Study the drawing (mm; zero at the part's minimum x, y, z) and answer. A direction names the side the tool comes from. Give positions to 0.01 mm unless a question says otherwise; leave off trailing zeros. Order: outer loops, then holes, each group sorted by start corner. A loop starts at its lowest first (then second) coordinate and runs counter-clockwise, first axis right, second up.
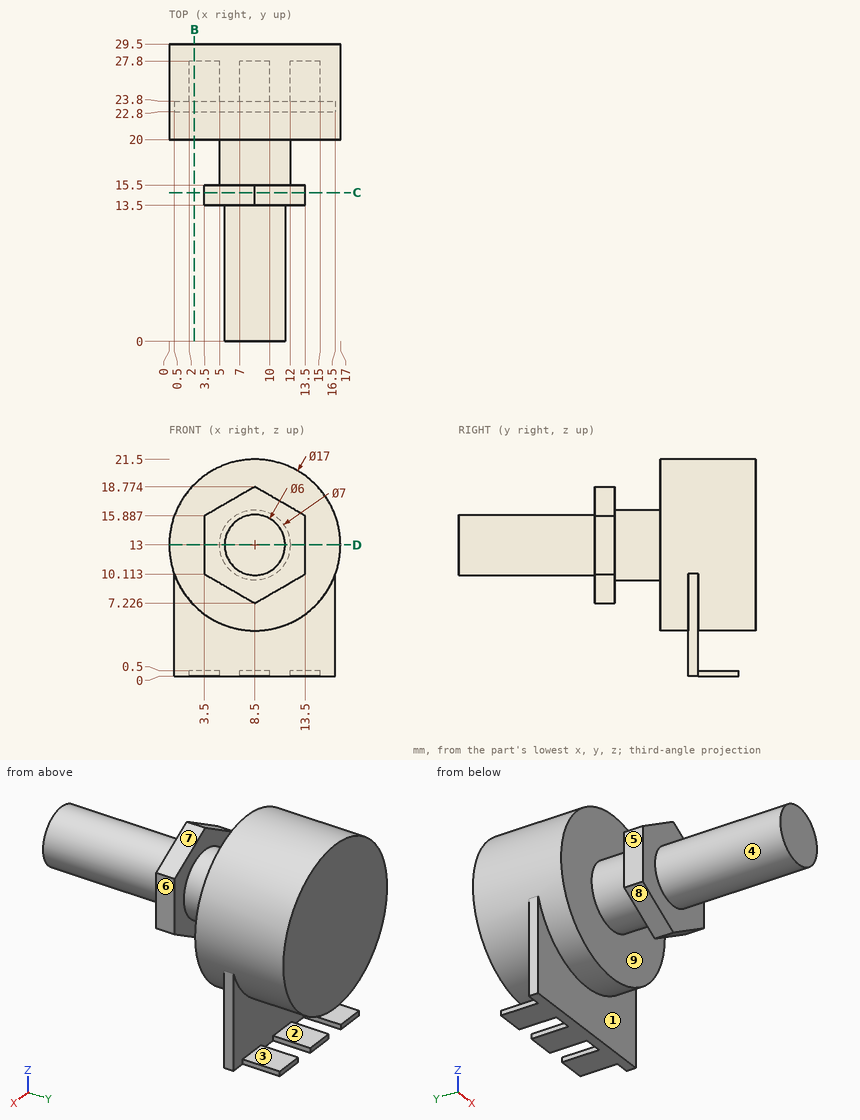
1) Find section D-D (z = 13). Write down the section's boundary in (x, y).
Geometry says:
outline: (0, 20) - (5, 20) - (5, 15.5) - (3.5, 15.5) - (3.5, 13.5) - (5.5, 13.5) - (5.5, 0) - (11.5, 0) - (11.5, 13.5) - (13.5, 13.5) - (13.5, 15.5) - (12, 15.5) - (12, 20) - (17, 20) - (17, 29.5) - (0, 29.5) - close
2) For a pull along Z with two mould halves and no side action, classify the marked faces 1, 2, 3 and 4 as +Z half, -Z half, draft (parallel to the pull), parting line (faces both ways), or undercut.
Geometry says:
face 1: draft
face 2: undercut
face 3: undercut
face 4: parting line
3) Find section C-C (y = 14.75). Write down the section's boundary in (x, z).
Geometry says:
outline: (3.5, 10.11) - (8.5, 7.23) - (13.5, 10.11) - (13.5, 15.89) - (8.5, 18.77) - (3.5, 15.89) - close
4) Straight lines are drawn through the part: probe 1 along Y at (x, z) = (11, 9.25); probe 2 along Y at (x, z) = (8.75, 19.75); probe 3 along Z at (x, y) = (2.75, 26). For each, find the intervals that lie inside material, in ascending order.
Geometry says:
probe 1: y = 13.5 to 15.5, 20 to 29.5
probe 2: y = 20 to 29.5
probe 3: z = 0 to 0.5, 6.74 to 19.26
5) Find section B-B (x = 2.5). Write down the section's boundary in (y, z).
Geometry says:
outline: (20, 6.98) - (22.8, 6.98) - (22.8, 0) - (27.8, 0) - (27.8, 0.5) - (23.8, 0.5) - (23.8, 6.98) - (29.5, 6.98) - (29.5, 19.02) - (20, 19.02) - close
6) A tool of negligible diameter and unlimited length cuts with its end or side. For the marked faces 5, 6, 7, 8 and 9, from which of +Z, -Z, +X, -X, +Y, -Y can it reach the whole face along a straight path? Write none if from no direction.
Geometry says:
face 5: +Z, -Z, -X, -Y
face 6: +Z, -Z, +X, -Y
face 7: +Z, +X, -Y
face 8: -Z, -X, -Y
face 9: none
7) Given P1, Ø0.6, axis at x = 13, z = 0.5, coming from the +Y side; P2, Ø0.8, axis at y = 23.5, z = 4.5, coming from the +X side; P3, Ø5, axis at x = 6, z = 6.5, coming from the -Y side; P4, Ø2, axis at x = 8.5, z = 13.5, coming from the -Y side, each flat-ended and moving along its own axis, determine where each tip first touches the part or whether it passes through.
Geometry says:
P1: stops at y = 27.8
P2: stops at x = 16.5
P3: stops at y = 13.5
P4: stops at y = 0
